Autodesk Inventor part; units mm, degrees
ref_plane "YZ Plane" through (0, 0, 0) normal (1, 0, 0) x (0, 1, 0)
ref_plane "XZ Plane" through (0, 0, 0) normal (0, 1, 0) x (-1, 0, 0)
ref_plane "XY Plane" through (0, 0, 0) normal (0, 0, 1) x (1, 0, 0)
sketch "草圖1" plane through (0, 0, 0) normal (0, 0, 1) x (1, 0, 0)
  circle A0 centre (0, 0) radius 1.6
  dimension "d0" = 3.2
extrude "擠出1" add sketch "草圖1" along normal blind 10
sketch "草圖2" plane through (0, 0, 10) normal (0, 0, 1) x (1, 0, 0)
  line L0 (2.5, -0.1) -> (-2.5, -0.1)
  line L1 (-2.5, -0.1) -> (-2.5, 0.1)
  line L2 (-2.5, 0.1) -> (2.5, 0.1)
  line L3 (2.5, 0.1) -> (2.5, -0.1)
  line L4 (2.5, -0.1) -> (-2.5, 0.1) construction
  line L5 (-2.5, -0.1) -> (2.5, 0.1) construction
  point P0 (0, 0)
  dimension "d3" = 5
  dimension "d4" = 0.2
sketch "草圖3" plane through (0, 0, 10) normal (0, 0, 1) x (1, 0, 0)
  circle A0 centre (0, 0) radius 1.6
extrude "擠出2" add sketch "草圖3" along normal blind 8 draft -5
extrude "擠出3" cut sketch "草圖2" along normal through all
fillet "圓角1" radius 1.6 1 edges at (-1.6, 0, 0)
properties part number "PMECAD_LEGOmini_FlagFrame" material "松木、赤松"
CAD build for the part. Positions are in the model's coordinates, mm. A direction names the side the tool comes from. Round coordinates to 2 decimals unless told otherwise and drop trailing zeros. Loops run counter-clockwise (first coordinate to the right, second up) from the corner with the lowest first, then second, coordinate; pieces in that order, holes last. Notation, with made-up numbers: (31.5, 79) - (45.5, 79) arc R26 cw to (45.5, 97) - close; hole circle Ø6 at (14, -0.75). An arc over 180 degrees is marked (long way). Return JSON: item names as keys, results as strings. Group by question number.
Q1. Drill centre lines: line 1 along Y through (x, z) = (-1.1, 13); line 2 along X through (y, z) = (0.5, 8); line 3 along Y through (x, z) = (-0.5, 10.5). Where is each one in solid material? Low to high. Write a range as [from, to].
Q2. Band-saw the part on A-A on x = 0. Give the cut face in (y, z).
Q3. Flat gauge pins, fed straight in: pin 1 Ø1.5 at (x, z) = (0, 11) entering from +Y; pin 2 Ø1.5 at (y, z) = (0.5, 15) entering from -X; pin 3 Ø1.6 at (x, z) = (0, 12.5) entering from -Y. Where does each tip first touch, or does it go through?
Q4. Two-plate mould, pull along Y, no slides. Class faces 3 (the face through (0, -0.4, 18)), 4 (the face through (0, -0.1, 14)), 5 (the face through (-0.026, 1.255, 13.944)): +Y half, -Y half, draft (parallel to the pull), parting line (faces both ways), or undercut.
Q5. Tool access for faces 1 (the face through (0, 0.1, 14)), 2 (the face through (-1.27, 0.97, 5.74)): list every direction of +Z, -Z, +X, -X, +Y, -Y with a clear straight run to the whole face (end or side of a thin tool).
Solutions:
{
 "1": {"line 1": "y = [-0.76, -0.1], [0.1, 0.76]", "line 2": "x = [-1.52, 1.52]", "line 3": "y = [-1.47, -0.1], [0.1, 1.47]"},
 "2": {"outline": "(-1.6, 1.6) arc R1.6 ccw to (1.6, 1.6) - (1.6, 10) - (0.9, 18) - (0.1, 18) - (0.1, 10) - (-0.1, 10) - (-0.1, 18) - (-0.9, 18) - (-1.6, 10) - close"},
 "3": {"pin 1": "stops at y = 1.58", "pin 2": "stops at x = -1.21", "pin 3": "stops at y = -1.45"},
 "4": {"face 3": "draft", "face 4": "undercut", "face 5": "+Y half"},
 "5": {"face 1": "+Z, +X, -X", "face 2": "+Z, -Z"}
}
